from build123d import *

# Parameters (mm, degrees)
F0_W     = 127
F0_H     = 165.1
F0_R     = 15.875
F1_DEPTH = 25.4
F2_R     = 3.175
F3_DEPTH = 6.35
F4_DEPTH = 25.4
F6_DEPTH = 25.4
F7_W     = 32.5129989862
F7_H     = 30.6838553727
F8_DEPTH = 127


with BuildPart() as f1:
    # F0 (on Front) → F1 (new body)
    with BuildSketch(Plane.XZ):
        Rectangle(F0_W, F0_H)
        with Locations((-38.1, 57.15)):
            Circle(F0_R, mode=Mode.SUBTRACT)
    extrude(amount=-F1_DEPTH)

    # F2 (on face) → F3 (cut)
    with BuildSketch(Plane.XZ):
        Polygon((63.5, -36.83), (-63.5, -44.45), (-63.5, -82.55), (63.5, -82.55), align=None)
        with Locations((-40.2505024661, -71.1942345153)):
            Circle(F2_R, mode=Mode.SUBTRACT)
        with Locations((-50.0621663703, -56.3665694452)):
            Circle(F2_R, mode=Mode.SUBTRACT)
        with Locations((-32.2821663703, -55.2997694452)):
            Circle(F2_R, mode=Mode.SUBTRACT)
        with Locations((-50.0621663703, -56.3665694452)):
            Circle(F2_R)
        with Locations((-32.2821663703, -55.2997694452)):
            Circle(F2_R)
        with Locations((-40.2505024661, -71.1942345153)):
            Circle(F2_R)
    extrude(amount=-F3_DEPTH, mode=Mode.SUBTRACT)

    # F2 (on face) → F4 (cut)
    with BuildSketch(Plane.XZ):
        with Locations((-50.0621663703, -56.3665694452)):
            Circle(F2_R)
        with Locations((-32.2821663703, -55.2997694452)):
            Circle(F2_R)
        with Locations((-40.2505024661, -71.1942345153)):
            Circle(F2_R)
    extrude(amount=-F4_DEPTH, mode=Mode.SUBTRACT)

    # F5 (on face) → F6 (cut)
    with BuildSketch(Plane.XZ.offset(-6.35)):
        Polygon((-61.214, -82.55), (-63.5, -44.45), (-63.5, -82.55), align=None)
    extrude(amount=-F6_DEPTH, mode=Mode.SUBTRACT)

    # F7 (on face) → F8 (join)
    with BuildSketch(Plane.XZ):
        with BuildLine():
            Line((-16.2564994931, 0), (16.2564994931, 0))
            ThreePointArc((16.2564994931, 0), (20.7466275537, 1.8598719395), (22.6064994931, 6.35))
            Line((22.6064994931, 6.35), (22.6064994931, 37.0338553727))
            ThreePointArc((22.6064994931, 37.0338553727), (20.7466275537, 41.5239834332), (16.2564994931, 43.3838553727))
            Line((16.2564994931, 43.3838553727), (-16.2564994931, 43.3838553727))
            ThreePointArc((-16.2564994931, 43.3838553727), (-20.7466275537, 41.5239834332), (-22.6064994931, 37.0338553727))
            Line((-22.6064994931, 37.0338553727), (-22.6064994931, 6.35))
            ThreePointArc((-22.6064994931, 6.35), (-20.7466275537, 1.8598719395), (-16.2564994931, 0))
        make_face()
        with Locations((0, 21.6919276863)):
            Rectangle(F7_W, F7_H, mode=Mode.SUBTRACT)
    extrude(amount=-F8_DEPTH)


solid = f1.part
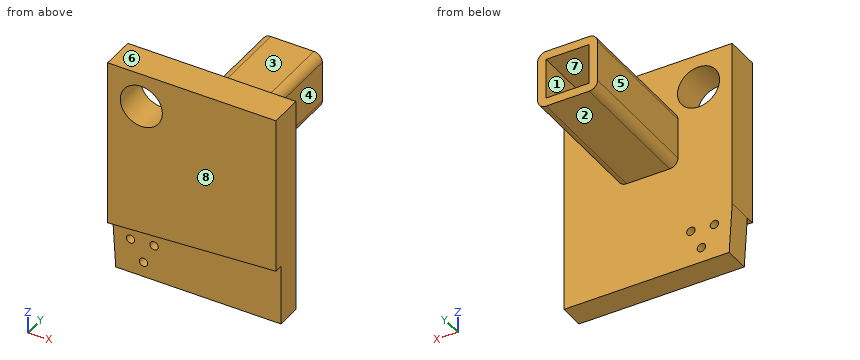
Check sheet for the modelled part. Datum: model origin and axes. Units: mm. Face numbers are marked on the shaded views. A direction names the side the tool comes from. Round coordinates to 2 decimals unless told otherwise and drop trailing zeros. Order: outer loops, then holes, each group sorted by start corner. A loop starts at its lowest first (then second) coordinate and runs counter-clockwise, first axis right, second up. Notation, with made-up numbers: M 38,43 L 84,43 A11 ccw 84,57 Z; hole C 31.25,-15 d3. An arc over 180 degrees is marked long. One line per item, written item: value. Start each with the question number.
1. Section check A-A on z = 57.15. Enter the section's corners in (x, y) (3 decimals), and give its area (3 significant figures).
2. Release check for a two-part mould opening along Z. For the marked faces 6, 7 and 8 record: released by +Z, released by -Z, zero draft, split by the parting line, or undercut.
3. Section check B-B on y = 113. Enter the section's corners in (x, z), and give its area (3 significant figures).
4. Scan lines: line 1 along X through (y, z) = (42.5, 18); line 2 along X through (y, z) = (8, 57); line 3 along Y through (x, z) = (-49, 74). Record each from-to range of solid material in increasing order.
5. Section check D-D on x = -50.5. Enter the section's corners in (y, z).
6. Section check C-C on x = -6. Enter the section's corners in (y, z).
7. Gauge pin test, flat ends, axial feed: P1, Ø15.5, axis at y = 100.5, z = 27.5, coming from the +X side; P2, Ø24.5, axis at y = 99.5, z = 23, coming from the -X side; P3, Ø16.5, axis at x = -6.5, y = 75, coming from the -Z side. Record the tip position at first contact, or that the pin passes through.
8. Access from +Z, -Z, +X, -X, +Y, -Y to the whole of each face (thin tool, end or side, straight path). Record for the marked faces 1, 2, 3, 4 and 5.
Results found:
1. outline: M -63.5,0 L -53.975,0 L -53.975,25.4 L -63.5,25.4 Z; M -22.225,0 L 63.5,0 L 63.5,25.4 L -22.225,25.4 Z
1. area: 2,420 mm^2
2. face 6: released by +Z
2. face 7: undercut
2. face 8: zero draft
3. outline: M -22.61,6.35 A6.35 ccw -16.26,0 L 16.26,0 A6.35 ccw 22.61,6.35 L 22.61,37.03 A6.35 ccw 16.26,43.38 L -16.26,43.38 A6.35 ccw -22.61,37.03 Z; hole M -16.26,6.35 L 16.26,6.35 L 16.26,37.03 L -16.26,37.03 Z
3. area: 929 mm^2
4. line 1: -22.61 to -16.26, 16.26 to 22.61
4. line 2: -63.5 to -53.97, -22.23 to 63.5
4. line 3: 0 to 25.4
5. outline: M 0,-43.67 L 6.35,-43.67 L 6.35,-53.22 L 25.4,-53.22 L 25.4,47.24 L 0,47.24 Z; M 0,67.06 L 25.4,67.06 L 25.4,82.55 L 0,82.55 Z; M 6.35,-82.55 L 25.4,-82.55 L 25.4,-59.51 L 6.35,-59.51 Z
6. outline: M 0,-41 L 6.35,-41 L 6.35,-82.55 L 25.4,-82.55 L 25.4,0 L 127,0 L 127,6.35 L 25.4,6.35 L 25.4,37.03 L 127,37.03 L 127,43.38 L 25.4,43.38 L 25.4,82.55 L 0,82.55 Z
7. P1: x = 22.61
7. P2: x = -22.61
7. P3: z = 0
8. face 1: +Y
8. face 2: -Z, +X, -X, +Y
8. face 3: +Z, +X, -X, +Y
8. face 4: +Z, -Z, +X, +Y
8. face 5: +Z, -Z, -X, +Y
